Source: CAD feature listing. Evaluate the final solid. Frame: model axes, mm. A direction names the side the tool comes from. Round coordinates to 2 decimals unless told otherwise and drop trailing zeros. Order: outer loops, then holes, each group sorted by start corner. A loop starts at its lowest first (then second) coordinate and runs counter-clockwise, first axis right, second up. Notation, with made-up numbers: (-16.5, -8) -> (16.5, -8) arc R36 ccw to (16.5, 28) -> close; hole circle Ø9 at (23.25, -22). An arc over 180 degrees is marked (long way). Answer as CSV lines item,"result". Start each with the question number.
(1) Line query: line 1 along Z through (x, y) = (25, 1.65); line 2 along X through (y, z) = (4.5, 0) (3 decimals); line 3 along Y through (x, z) = (8, -4). Output: solid intervals per line, ascending. Write a range as from..to.
(2) Section query A-A (z = 0). Output: boundary loops of the cut face in (x, y) (3 decimals), plus the area to 3 significant figures.
(3) Section query D-D (y = 1.25). Output: boundary loops of the cut face in (x, z) (3 decimals).
(4) Contact query for flat-ended pins moving along their axis: P1, Ø6.5, axis at x = -5.5, z = -1.5, coming from the -Y side; P2, Ø4, axis at x = 25, z = -15.1, coming from the +Y side. Output: stop coordinate, or through.
(5) Section query B-B (x = 25). Output: boundary loops of the cut face in (y, z), plus the area to 3 significant figures.
(6) Set-up query: faces 1 (the cylindrical face through (25.901, 5.796, -12.237)), 2 (the cylindrical face through (-19.094, 4.437, 0.42)), 3 (the flat face through (2.6, 7, 7.2)). Return all of +Z, -Z, +X, -X, +Y, -Y with unobstructed straight access to the full face (end or side cutting, diameter ignored); none if empty.
(7) Section query C-C (y = 7.75). Output: boundary loops of the cut face in (x, z), plus the area to 3 significant figures.
(8) Pull-direction query (Z, two-part tool) for faces 4 (the cylindrical face through (24.9, 1.2, -13.5)), 5 (the flat face through (12, 9, 0)), 6 (the cylindrical face through (30.797, 4.437, -17.958)); classes: +Z half, -Z half, draft (parallel to the pull), parting line (faces both ways), or undercut.
```python
from build123d import *

# Parameters (mm, degrees)
SKIZZE1_R                       = 1.6
SKIZZE1_R_2                     = 11.075
AUFSATZ_LINEAR_AUSTRAGEN1_DEPTH = 7
SKIZZE3_R                       = 7.5
AUFSATZ_LINEAR_AUSTRAGEN2_DEPTH = 2
SKIZZE4_R                       = 3
SCHNITT_LINEAR_AUSTRAGEN1_DEPTH = 6.5
VERRUNDUNG4_R                   = 4


with BuildPart() as part:
    # Skizze1 → Aufsatz-Linear austragen1 (new body)
    with BuildSketch(Plane(origin=(0, 0, 0), x_dir=(1, 0, 0), z_dir=(0, 1, 0))):
        with BuildLine():
            Line((0, 19.098593171), (32, 19.098593171))
            Line((32, 19.098593171), (32, -19.098593171))
            Line((32, -19.098593171), (0, -19.098593171))
            ThreePointArc((0, -19.098593171), (-19.098593171, 0), (0, 19.098593171))
        make_face()
        with Locations(Location((25, -15.098593171, 0), (0, 0, 270))):
            Circle(SKIZZE1_R, mode=Mode.SUBTRACT)
        with Locations(Location((25, 15.098593171, 0), (0, 0, 90))):
            Circle(SKIZZE1_R, mode=Mode.SUBTRACT)
        with Locations(Location((0, 0, 0), (0, 0, 270))):
            Circle(SKIZZE1_R_2, mode=Mode.SUBTRACT)
    extrude(amount=AUFSATZ_LINEAR_AUSTRAGEN1_DEPTH)

    # Skizze3 → Aufsatz-Linear austragen2 (add)
    with BuildSketch(Plane(origin=(0, 7, 0), x_dir=(1, 0, 0), z_dir=(0, 1, 0))):
        with BuildLine():
            Line((0, 19.098593171), (32, 19.098593171))
            Line((32, 19.098593171), (32, -19.098593171))
            Line((32, -19.098593171), (0, -19.098593171))
            ThreePointArc((0, -19.098593171), (-19.098593171, 0), (0, 19.098593171))
        make_face()
        with Locations(Location((0, 0, 0), (0, 0, 270))):
            Circle(SKIZZE3_R, mode=Mode.SUBTRACT)
    extrude(amount=AUFSATZ_LINEAR_AUSTRAGEN2_DEPTH)

    # Skizze4 → Schnitt-Linear austragen1 (cut)
    with BuildSketch(Plane(origin=(0, 9, 0), x_dir=(1, 0, 0), z_dir=(0, 1, 0))):
        with Locations(Location((25, 15.098593171, 0), (0, 0, 270))):
            Circle(SKIZZE4_R)
        with Locations(Location((25, -15.098593171, 0), (0, 0, 270))):
            Circle(SKIZZE4_R)
    extrude(amount=-SCHNITT_LINEAR_AUSTRAGEN1_DEPTH, mode=Mode.SUBTRACT)

    # Verrundung4
    verrundung4_edges = [part.edges().sort_by_distance(p)[0] for p in [
        (32, 4.5, -19.098593171),
        (32, 4.5, 19.098593171),
    ]]
    fillet(verrundung4_edges, radius=VERRUNDUNG4_R)


solid = part.part
```
Answer block:
1,line 1,"-19.1..-16.7, -13.5..13.5, 16.7..19.1"
1,line 2,"-19.099..-11.075, 11.075..32"
1,line 3,"7..9"
2,outline,"(-19.099, 0) -> (-11.075, 0) -> (-11.075, 7) -> (-7.5, 7) -> (-7.5, 9) -> (-19.099, 9) -> close; (7.5, 7) -> (11.075, 7) -> (11.075, 0) -> (32, 0) -> (32, 9) -> (7.5, 9) -> close"
2,area,"275 mm2"
3,outline,"(0, -19.099) -> (28, -19.099) arc R4 ccw to (32, -15.099) -> (32, 15.099) arc R4 ccw to (28, 19.099) -> (0, 19.099) arc R19.099 ccw to start; hole circle Ø22.15 at (0, 0); hole circle Ø3.2 at (25, -15.099); hole circle Ø3.2 at (25, 15.099)"
4,P1,"y = 7"
4,P2,"y = 2.5"
5,outline,"(0, -19.1) -> (9, -19.1) -> (9, -18.1) -> (2.5, -18.1) -> (2.5, -16.7) -> (0, -16.7) -> close; (0, -13.5) -> (2.5, -13.5) -> (2.5, -12.1) -> (9, -12.1) -> (9, 12.1) -> (2.5, 12.1) -> (2.5, 13.5) -> (0, 13.5) -> close; (0, 16.7) -> (2.5, 16.7) -> (2.5, 18.1) -> (9, 18.1) -> (9, 19.1) -> (0, 19.1) -> close"
5,area,"250 mm2"
6,face 1,"+Y"
6,face 2,"-X, +Y, -Y"
6,face 3,"-Y"
7,outline,"(0, -19.1) -> (28, -19.1) arc R4 ccw to (32, -15.1) -> (32, 15.1) arc R4 ccw to (28, 19.1) -> (0, 19.1) arc R19.1 ccw to start; hole circle Ø15 at (0, 0); hole circle Ø6 at (25, -15.1); hole circle Ø6 at (25, 15.1)"
7,area,"1,560 mm2"
8,face 4,"undercut"
8,face 5,"draft"
8,face 6,"-Z half"
